Can you work these out from the model? Positions are in its coordinate system, mm. A direction names the side the tool comes from. Give positions to 0.01 mm unless a question says otherwise; leave off trailing zeros. Order: outer loops, then holes, each group sorted by start corner. A loop starts at its lowest first (then second) coordinate and runs counter-clockwise, first axis right, second up. Notation, with made-up numbers: (2.5, 51) -> (41.5, 51) arc R17 ccw to (41.5, 84) -> close; hole circle Ø10 at (3, -0.75). An arc over 180 degrees is marked (long way). Answer as CSV lines item,"result".
```python
from build123d import *

# Parameters (mm, degrees)
EXTRUDE1_DEPTH                       = 32.5
SKETCH3_W                            = 60
SKETCH3_H                            = 55
CUT_EXTRUDE1_DEPTH                   = 48.5
CUT_EXTRUDE1_DEPTH_BACK              = 650.5
SKETCH4_W                            = 25.25
SKETCH4_H                            = 66
CUT_EXTRUDE2_DEPTH                   = 35
F_8_CLEARANCE_HOLE1_D                = 4.4958
LPATTERN1_COUNT                      = 7
LPATTERN1_PITCH                      = 90
TAPPED_HOLE_FOR_8_32_HELICOIL2_D     = 4.3942
TAPPED_HOLE_FOR_8_32_HELICOIL2_DEPTH = 11.1252
TAPPED_HOLE_FOR_8_32_HELICOIL2_TIP   = 1.320150866
TAPPED_HOLE_FOR_8_32_HELICOIL6_D     = 4.3942
TAPPED_HOLE_FOR_8_32_HELICOIL6_DEPTH = 11.1252
TAPPED_HOLE_FOR_8_32_HELICOIL6_TIP   = 1.320150866
TAPPED_HOLE_FOR_8_32_HELICOIL3_D     = 4.3942
TAPPED_HOLE_FOR_8_32_HELICOIL4_D     = 4.3942
SKETCH35_W                           = 83.352933337
SKETCH35_H                           = 26
SKETCH35_H_2                         = 10
EXTRUDE18_DEPTH                      = 206.779133429
TAPPED_HOLE_FOR_8_32_HELICOIL5_D     = 4.3942
CUT_EXTRUDE4_DEPTH                   = 66
CHAMFER1_SIZE                        = 10
SKETCH38_W                           = 17.65
SKETCH38_H                           = 15
CUT_EXTRUDE5_DEPTH                   = 66
CHAMFER2_SIZE                        = 10
CUT_EXTRUDE13_START                  = 32.5
SKETCH40_W                           = 12.75
SKETCH40_H                           = 56
CUT_EXTRUDE13_DEPTH                  = 3
CUT_EXTRUDE14_START                  = -32.5
SKETCH40_3_W                         = 12.75
SKETCH40_3_H                         = 56
CUT_EXTRUDE14_DEPTH                  = 3
SKETCH42_W                           = 91.864816585
SKETCH42_H                           = 689.904772547
SKETCH42_W_2                         = 59
SKETCH42_H_2                         = 10
SKETCH42_W_3                         = 65
SKETCH42_H_3                         = 35
CUT_EXTRUDE15_DEPTH                  = 3
FILLET2_R                            = 2.5


with BuildPart() as part:
    # Sketch2 → Extrude1 (new body, symmetric)
    with BuildSketch(Plane.XY):
        Polygon((170.229133429, 47.5), (170.229133429, -47.5), (159.529133429, -87.432943641), (159.529133429, -514.567056359), (170.229133429, -554.5), (170.229133429, -649.5), (205.779133429, -649.5), (205.779133429, 47.5), align=None)
    extrude(amount=EXTRUDE1_DEPTH, both=True)

    # Sketch3 → Cut-Extrude1 (cut, two sides)
    with BuildSketch(Plane(origin=(0, 0, 0), x_dir=(1, 0, 0), z_dir=(0, 1, 0))) as cut_extrude1_sk:
        with Locations((170.779133429, 0)):
            Rectangle(SKETCH3_W, SKETCH3_H)
    extrude(amount=CUT_EXTRUDE1_DEPTH, mode=Mode.SUBTRACT)
    extrude(cut_extrude1_sk.sketch, amount=-CUT_EXTRUDE1_DEPTH_BACK, mode=Mode.SUBTRACT)

    # Sketch4 → Cut-Extrude2 (cut, symmetric)
    with BuildSketch(Plane.XY):
        with Locations((196.404133429, -262.7)):
            Rectangle(SKETCH4_W, SKETCH4_H)
    extrude(amount=CUT_EXTRUDE2_DEPTH, both=True, mode=Mode.SUBTRACT)

    # 8 Clearance Hole1 (through all)
    with Locations(Plane(origin=(205.779133429, -77.5, -7.728), x_dir=(0, 1, 0), z_dir=(1, 0, 0))):
        with Locations((0, 0)):
            f_8_clearance_hole1 = Hole(F_8_CLEARANCE_HOLE1_D / 2)

    # LPattern1: 8 Clearance Hole1 ×7, 2 skipped
    with Locations(*[(0, -i * LPATTERN1_PITCH, 0) for i in range(1, LPATTERN1_COUNT) if i not in (2, 6)]):
        add(f_8_clearance_hole1, mode=Mode.SUBTRACT)

    # Tapped Hole for _8-32 Helicoil2
    with Locations(Plane(origin=(194.579133429, -27.5, 32.5), x_dir=(1, 0, 0), z_dir=(0, 0, 1))):
        with Locations((0, 0), (0, -15), (0, -75), (0, -90), (0, -285), (0, -300), (0, -558.7), (0, -573.7)):
            Hole(TAPPED_HOLE_FOR_8_32_HELICOIL2_D / 2, depth=TAPPED_HOLE_FOR_8_32_HELICOIL2_DEPTH)
            with Locations((0, 0, -(TAPPED_HOLE_FOR_8_32_HELICOIL2_DEPTH + TAPPED_HOLE_FOR_8_32_HELICOIL2_TIP / 2))):  # 118° drill point
                Cone(0, TAPPED_HOLE_FOR_8_32_HELICOIL2_D / 2, TAPPED_HOLE_FOR_8_32_HELICOIL2_TIP, mode=Mode.SUBTRACT)

    # Tapped Hole for _8-32 Helicoil6
    with Locations(Plane(origin=(0, 0, -32.5), x_dir=(-1, 0, 0), z_dir=(0, 0, -1))):
        with Locations((-194.579133429, -27.5), (-194.579133429, -42.5), (-194.579133429, -102.5), (-194.579133429, -117.5), (-194.579133429, -312.5), (-194.579133429, -327.5), (-194.579133429, -586.2), (-194.579133429, -601.2)):
            Hole(TAPPED_HOLE_FOR_8_32_HELICOIL6_D / 2, depth=TAPPED_HOLE_FOR_8_32_HELICOIL6_DEPTH)
            with Locations((0, 0, -(TAPPED_HOLE_FOR_8_32_HELICOIL6_DEPTH + TAPPED_HOLE_FOR_8_32_HELICOIL6_TIP / 2))):  # 118° drill point
                Cone(0, TAPPED_HOLE_FOR_8_32_HELICOIL6_D / 2, TAPPED_HOLE_FOR_8_32_HELICOIL6_TIP, mode=Mode.SUBTRACT)

    # Tapped Hole for _8-32 Helicoil3 (through all)
    with Locations(Plane(origin=(205.779133429, 0, 0), x_dir=(0, 0, -1), z_dir=(1, 0, 0))):
        with Locations((-17.8, -317.5), (17.8, -317.5), (-17.8, -332.5), (17.8, -332.5)):
            Hole(TAPPED_HOLE_FOR_8_32_HELICOIL3_D / 2)

    # Tapped Hole for _8-32 Helicoil4 (through all)
    with Locations(Plane(origin=(174.529133429, -239.7, 32.5), x_dir=(1, 0, 0), z_dir=(0, 0, 1))):
        with Locations((0, 0), (0, -46)):
            Hole(TAPPED_HOLE_FOR_8_32_HELICOIL4_D / 2)

    # Sketch35 → Extrude18 (cut, through all)
    with BuildSketch(Plane(origin=(0, 0, 0), x_dir=(0, 0, -1), z_dir=(1, 0, 0))):
        with Locations((-1.322638192, 36.5)):
            Rectangle(SKETCH35_W, SKETCH35_H)
        with Locations((-1.322638192, -646.5)):
            Rectangle(SKETCH35_W, SKETCH35_H_2)
    extrude(amount=EXTRUDE18_DEPTH, mode=Mode.SUBTRACT)

    # Tapped Hole for _8-32 Helicoil5 (through all)
    with Locations(Plane(origin=(205.779133429, 19.5, 17.5), x_dir=(0, 1, 0), z_dir=(1, 0, 0))):
        with Locations((0, 0), (0, -35)):
            Hole(TAPPED_HOLE_FOR_8_32_HELICOIL5_D / 2)

    # Sketch37 → Cut-Extrude4 (cut, through all)
    with BuildSketch(Plane(origin=(0, 0, -32.5), x_dir=(-1, 0, 0), z_dir=(0, 0, -1))):
        Polygon((-200.779133429, -641.5), (-170.229133429, -641.5), (-170.229133429, -609.356521994), (-170.229133429, -600.5), (-178.279133429, -600.5), (-178.279133429, -614), (-200.779133429, -614), align=None)
    extrude(amount=-CUT_EXTRUDE4_DEPTH, mode=Mode.SUBTRACT)

    # Chamfer1
    chamfer1_edges = [part.edges().sort_by_distance(p)[0] for p in [
        (178.279133429, -614, -30),
        (178.279133429, -614, 30),
    ]]
    chamfer(chamfer1_edges, length=CHAMFER1_SIZE)

    # Sketch38 → Cut-Extrude5 (cut, through all)
    with BuildSketch(Plane.XY.offset(32.5)):
        with Locations((179.054133429, 16)):
            Rectangle(SKETCH38_W, SKETCH38_H)
    extrude(amount=-CUT_EXTRUDE5_DEPTH, mode=Mode.SUBTRACT)

    # Chamfer2
    chamfer2_edges = [part.edges().sort_by_distance(p)[0] for p in [
        (187.879133429, 23.5, 30),
        (187.879133429, 23.5, -30),
    ]]
    chamfer(chamfer2_edges, length=CHAMFER2_SIZE)

    # Sketch40 → Cut-Extrude13 (cut)
    with BuildSketch(Plane.XY.offset(CUT_EXTRUDE13_START)):
        Polygon((134.931335664, 87.372466397), (210.779133429, 87.372466397), (210.779133429, -20), (183.779133429, -20), (183.779133429, -50), (210.779133429, -50), (210.779133429, -95), (183.779133429, -95), (183.779133429, -125), (210.779133429, -125), (210.779133429, -305), (183.779133429, -305), (183.779133429, -340), (210.779133429, -340), (210.779133429, -578.7), (183.779133429, -578.7), (183.779133429, -616.252685753), (134.931335664, -616.252685753), align=None)
        with Locations((177.404133429, -262.7)):
            Rectangle(SKETCH40_W, SKETCH40_H, mode=Mode.SUBTRACT)
    extrude(amount=-CUT_EXTRUDE13_DEPTH, mode=Mode.SUBTRACT)

    # Sketch40_3 → Cut-Extrude14 (cut)
    with BuildSketch(Plane.XY.offset(CUT_EXTRUDE14_START)):
        Polygon((134.931335664, 87.372466397), (210.779133429, 87.372466397), (210.779133429, -20), (183.779133429, -20), (183.779133429, -50), (210.779133429, -50), (210.779133429, -95), (183.779133429, -95), (183.779133429, -125), (210.779133429, -125), (210.779133429, -305), (183.779133429, -305), (183.779133429, -340), (210.779133429, -340), (210.779133429, -578.7), (183.779133429, -578.7), (183.779133429, -616.252685753), (134.931335664, -616.252685753), align=None)
        with Locations((177.404133429, -262.7)):
            Rectangle(SKETCH40_3_W, SKETCH40_3_H, mode=Mode.SUBTRACT)
    extrude(amount=CUT_EXTRUDE14_DEPTH, mode=Mode.SUBTRACT)

    # Sketch42 → Cut-Extrude15 (cut)
    with BuildSketch(Plane(origin=(205.779133429, 0, 0), x_dir=(0, 0, -1), z_dir=(1, 0, 0))):
        with Locations((-0.915268581, -304.741083254)):
            Rectangle(SKETCH42_W, SKETCH42_H)
        with Locations((0, 18.5)):
            Rectangle(SKETCH42_W_2, SKETCH42_H_2, mode=Mode.SUBTRACT)
        with Locations((0, -322.5)):
            Rectangle(SKETCH42_W_3, SKETCH42_H_3, mode=Mode.SUBTRACT)
        with Locations((0, -636.5)):
            Rectangle(SKETCH42_W_3, SKETCH42_H_2, mode=Mode.SUBTRACT)
    extrude(amount=-CUT_EXTRUDE15_DEPTH, mode=Mode.SUBTRACT)

    # Fillet2
    fillet2_edges = [part.edges().sort_by_distance(p)[0] for p in [
        (200.779133429, -614, -30),
        (200.779133429, -614, 30),
        (183.779133429, -229.7, -28.5),
        (183.779133429, -295.7, -28.5),
        (183.779133429, -295.7, 28.5),
        (183.779133429, -229.7, 28.5),
    ]]
    fillet(fillet2_edges, radius=FILLET2_R)


solid = part.part
```
Item 1: Imagine slicing it at A-A, the plane z = 9.5. Please give me the cut outline in (x, y), then the cut area to 3 significant figures.
Numbers:
outline,"(200.78, -641.5) -> (205.78, -641.5) -> (205.78, -631.5) -> (202.78, -631.5) -> (202.78, -340) -> (205.78, -340) -> (205.78, -305) -> (202.78, -305) -> (202.78, -295.7) -> (200.78, -295.7) -> close; (200.78, -229.7) -> (202.78, -229.7) -> (202.78, 13.5) -> (205.78, 13.5) -> (205.78, 23.5) -> (200.78, 23.5) -> close"
area,"1,360 mm²"
Item 2: For faces 4 (the flat face through (202.779, -106, 0)), 5 (the flat face through (200.779, -105, 0)), 6 (the flat face through (193, -35, -32.5)), which set-ups out of +Z, -Z, +X, -X, +Y, -Y let a thin tool reach every point of the face, with its end or its side?
Numbers:
face 4,"+Z, -Z, +X"
face 5,"-X, +Y, -Y"
face 6,"-Z, +X, -X, +Y, -Y"
Item 3: Please list where these lines run through material, in increasing order: line 1 along X through (y, z) = (-117, -29); line 2 along Z through (x, y) = (197, -425); line 3 along Z through (x, y) = (201.7, -167.5).
Numbers:
line 1,"x = 159.53 to 192.44, 196.72 to 202.78"
line 2,"z = -29.5 to -27.5, 27.5 to 29.5"
line 3,"z = -29.5 to -9.98, -5.48 to 29.5"
Item 4: We'd pull the mould along Z, two halves only. Please class faces 1 (the flat face through (180, -301, -27.5)), 2 (the flat face through (193, -110, -32.5)), 3 (the flat face through (203, -340, -2)): released by +Z, released by -Z, zero draft, split by the parting line, or undercut.
Numbers:
face 1,"undercut"
face 2,"released by -Z"
face 3,"zero draft"
Item 5: For pin 1 (3 mm diameter, centred on x = 182.5, y = -131.5, fed in from +Z); pin 2 (3 mm diameter, centred on y = -212.5, z = -23.5, fed in from -X); pin 3 (4 mm diameter, centred on y = -317.5, z = 17.8, fed in from +X); pin 4 (4 mm diameter, centred on x = 180.5, y = -306.5, fed in from -Z), each with a flat end and sliding along its axis, tell me the tip position at first contact or that it passes through.
Numbers:
pin 1,"stops at z = 29.5"
pin 2,"stops at x = 200.78"
pin 3,"passes through"
pin 4,"stops at z = -29.5"
